Check sheet for the modelled part. Datum: model origin and axes. Units: mm. A direction names the side the tool comes from. Give positions to 0.01 mm unless a question says otherwise; leave off trailing zeros. Write each loop counter-clockwise with the first axis right and the second up, starting at its lowest first coordinate (ties: lowest second). Pieces come first, ordered by that corner, then holes. Notation, with made-up numbers: (49.25, 11) -> (82.25, 11) arc R5 cw to (82.25, 19) -> close; hole circle Ø9 at (-3, 26). An arc over 180 degrees is marked (long way). Return JSON: item names as keys, results as strings.
from build123d import *

# Parameters (mm, degrees)
PLATE_SKETCH_W                 = 80
PLATE_SKETCH_H                 = 70
PLATE_EXTRUDE_DEPTH            = 15
HOLE_CUT_REACH                 = 57.227
HOLE_SKETCH_R                  = 5.5
HOLE_CUT_DIRECTION_2_REACH     = 57.227
FEMALE_FILLET_RADIUS           = 7.5
FEMALE_FILLET_LENGTH           = 70
GAP_CUT_DEPTH                  = 10
GAP_CUT_DEPTH_BACK             = 10
GAP_SKETCH_W                   = 15
GAP_SKETCH_H                   = 15
PIN_SUPPORT_EXTRUDE_DEPTH      = 10
PIN_SUPPORT_EXTRUDE_DEPTH_BACK = 10
PIN_SUPPORT_SKETCH_W           = 15
PIN_SUPPORT_SKETCH_H           = 15
PIN_EXTRUDE_REACH              = 74.629
PIN_SKETCH_R                   = 5.5
PIN_EXTRUDE_DIRECTION_2_REACH  = 74.629
MALE_FILLET_RADIUS             = 7.5
MALE_FILLET_LENGTH             = 20


with BuildPart() as part:
    # Plate Sketch → Plate Extrude (new body)
    with BuildSketch(Plane.XY):
        Rectangle(PLATE_SKETCH_W, PLATE_SKETCH_H)
    extrude(amount=-PLATE_EXTRUDE_DEPTH)

    # Hole Cut: up to this face of the body (flat: up to its plane)
    hole_cut_end = Plane(part.part.faces().sort_by_distance((0, 35, -7.5))[0])
    # Hole Sketch → Hole Cut (cut, up to the picked face)
    with BuildSketch(Plane(origin=(0, 0, 0), x_dir=(1, 0, 0), z_dir=(0, 1, 0)), mode=Mode.PRIVATE) as hole_cut_sk1:
        with Locations(Location((-32.5, 7.5, 0), (0, 0, 90))):
            Circle(HOLE_SKETCH_R)
    hole_cut_tool1 = split(extrude(hole_cut_sk1.sketch, amount=HOLE_CUT_REACH, mode=Mode.PRIVATE), bisect_by=hole_cut_end, keep=Keep.BOTH, mode=Mode.PRIVATE)
    add(hole_cut_tool1.solids().sort_by(Axis((-32.5, 0, -7.5), (0, 1, 0)))[0], mode=Mode.SUBTRACT)

    # Hole Cut direction 2: up to this face of the body (flat: up to its plane)
    hole_cut_direction_2_end = Plane(part.part.faces().sort_by_distance((0, -35, -7.5))[0])
    # Hole Sketch → Hole Cut direction 2 (cut, up to the picked face)
    with BuildSketch(Plane(origin=(0, 0, 0), x_dir=(1, 0, 0), z_dir=(0, 1, 0)), mode=Mode.PRIVATE) as hole_cut_direction_2_sk1:
        with Locations(Location((-32.5, 7.5, 0), (0, 0, 90))):
            Circle(HOLE_SKETCH_R)
    hole_cut_direction_2_tool1 = split(extrude(hole_cut_direction_2_sk1.sketch, amount=-HOLE_CUT_DIRECTION_2_REACH, mode=Mode.PRIVATE), bisect_by=hole_cut_direction_2_end, keep=Keep.BOTH, mode=Mode.PRIVATE)
    add(hole_cut_direction_2_tool1.solids().sort_by(Axis((-32.5, 0, -7.5), (0, -1, 0)))[0], mode=Mode.SUBTRACT)

    # Female Fillet: full round fillet: the end face becomes a half cylinder, R = half its width
    female_fillet_face = Plane((-40, 0, -7.5), x_dir=(0, -1, 0), z_dir=(-1, 0, 0))  # on the end face: x along it, z out of the body
    female_fillet_slab = female_fillet_face.offset(-FEMALE_FILLET_RADIUS / 2) * Box(FEMALE_FILLET_LENGTH, 2 * FEMALE_FILLET_RADIUS, FEMALE_FILLET_RADIUS, mode=Mode.PRIVATE)  # the body's end, R deep
    female_fillet_round = Plane((-32.5, 0, -7.5), x_dir=(-1, 0, 0), z_dir=(0, -1, 0)) * Cylinder(FEMALE_FILLET_RADIUS, FEMALE_FILLET_LENGTH, mode=Mode.PRIVATE)  # its axis R under the face
    add(female_fillet_slab - female_fillet_round, mode=Mode.SUBTRACT)

    # Gap Sketch → Gap Cut (cut, two sides: drawn at the far end of the back side and taken through both)
    with BuildSketch(Plane(origin=(0, 0, 0), x_dir=(1, 0, 0), z_dir=(0, 1, 0)).offset(-GAP_CUT_DEPTH_BACK)):
        with Locations((-32.5, 7.5)):
            Rectangle(GAP_SKETCH_W, GAP_SKETCH_H)
    extrude(amount=GAP_CUT_DEPTH + GAP_CUT_DEPTH_BACK, mode=Mode.SUBTRACT)

    # Pin Support Sketch → Pin Support Extrude (add, two sides: drawn at the far end of the back side and taken through both)
    with BuildSketch(Plane(origin=(0, 0, 0), x_dir=(1, 0, 0), z_dir=(0, 1, 0)).offset(-PIN_SUPPORT_EXTRUDE_DEPTH_BACK)):
        with Locations((47.5, 7.5)):
            Rectangle(PIN_SUPPORT_SKETCH_W, PIN_SUPPORT_SKETCH_H)
    extrude(amount=PIN_SUPPORT_EXTRUDE_DEPTH + PIN_SUPPORT_EXTRUDE_DEPTH_BACK)

    # Pin Extrude: up to this face of the body (flat: up to its plane)
    pin_extrude_end = Plane(part.part.faces().sort_by_distance((3.713685867, 35, -7.5))[0])
    # Pin Sketch → Pin Extrude (add, up to the picked face)
    with BuildSketch(Plane(origin=(0, 10, 0), x_dir=(1, 0, 0), z_dir=(0, 1, 0)), mode=Mode.PRIVATE) as pin_extrude_sk1:
        with Locations(Location((47.5, 7.5, 0), (0, 0, 90))):
            Circle(PIN_SKETCH_R)
    pin_extrude_tool1 = split(extrude(pin_extrude_sk1.sketch, amount=PIN_EXTRUDE_REACH, mode=Mode.PRIVATE), bisect_by=pin_extrude_end, keep=Keep.BOTH, mode=Mode.PRIVATE)
    add(pin_extrude_tool1.solids().sort_by(Axis((47.5, 10, -7.5), (0, 1, 0)))[0])

    # Pin Extrude direction 2: up to this face of the body (flat: up to its plane)
    pin_extrude_direction_2_end = Plane(part.part.faces().sort_by_distance((3.713685867, -35, -7.5))[0])
    # Pin Sketch → Pin Extrude direction 2 (add, up to the picked face)
    with BuildSketch(Plane(origin=(0, 10, 0), x_dir=(1, 0, 0), z_dir=(0, 1, 0)), mode=Mode.PRIVATE) as pin_extrude_direction_2_sk1:
        with Locations(Location((47.5, 7.5, 0), (0, 0, 90))):
            Circle(PIN_SKETCH_R)
    pin_extrude_direction_2_tool1 = split(extrude(pin_extrude_direction_2_sk1.sketch, amount=-PIN_EXTRUDE_DIRECTION_2_REACH, mode=Mode.PRIVATE), bisect_by=pin_extrude_direction_2_end, keep=Keep.BOTH, mode=Mode.PRIVATE)
    add(pin_extrude_direction_2_tool1.solids().sort_by(Axis((47.5, 10, -7.5), (0, -1, 0)))[0])

    # Male Fillet: full round fillet: the end face becomes a half cylinder, R = half its width
    male_fillet_face = Plane((55, 0, -7.5), x_dir=(0, 1, 0), z_dir=(1, 0, 0))  # on the end face: x along it, z out of the body
    male_fillet_slab = male_fillet_face.offset(-MALE_FILLET_RADIUS / 2) * Box(MALE_FILLET_LENGTH, 2 * MALE_FILLET_RADIUS, MALE_FILLET_RADIUS, mode=Mode.PRIVATE)  # the body's end, R deep
    male_fillet_round = Plane((47.5, 0, -7.5), x_dir=(1, 0, 0), z_dir=(0, 1, 0)) * Cylinder(MALE_FILLET_RADIUS, MALE_FILLET_LENGTH, mode=Mode.PRIVATE)  # its axis R under the face
    add(male_fillet_slab - male_fillet_round, mode=Mode.SUBTRACT)


solid = part.part
(1) Set-up check for faces 4 (the flat face through (40, 22, -7)), 5 (the cylindrical face through (42.047, 22.325, -6.784)), 6 (the cylindrical face through (42.047, -22.325, -6.784)): record each of +Z, -Z, +X, -X, +Y, -Y from which the full face is reachable in a straight line by a thin tool's end or side.
Reply:
{"face 4": "+Z, -Z, +Y", "face 5": "+Y", "face 6": "-Y"}
(2) Cross-section at C-C on x = -34. Enter the section's corners in (y, z), then the cut area to 3 significant figures.
Reply:
{"outline": "(-35, -14.85) -> (-10, -14.85) -> (-10, -12.79) -> (-35, -12.79) -> close; (-35, -2.21) -> (-10, -2.21) -> (-10, -0.15) -> (-35, -0.15) -> close; (10, -14.85) -> (35, -14.85) -> (35, -12.79) -> (10, -12.79) -> close; (10, -2.21) -> (35, -2.21) -> (35, -0.15) -> (10, -0.15) -> close", "area": "206 mm^2"}
(3) Cross-section at A-A on y = 13. Enter the section's corners in (x, z), then the cut area to 3 significant figures.
Reply:
{"outline": "(-32.5, -15) -> (40, -15) -> (40, 0) -> (-32.5, 0) arc R7.5 ccw to start; circle Ø11 at (47.5, -7.5); hole circle Ø11 at (-32.5, -7.5)", "area": "1,180 mm^2"}
(4) Depth check by flat-ended pin: pin 1 Ø7.5 at (y, z) = (22, -8) entering from +X; pin 2 Ø1.5 at (y, z) = (-5.5, -3.5) entering from -X. Enter the tip coordinate at first touch or a pass-through.
Reply:
{"pin 1": "x = 53", "pin 2": "x = -25"}
(5) Thickness scan on L1, parallel to X at y = -15, z = -7.5; L2, parallel to Z at x = -32.5, y = -24.75; L3, parallel to X at y = 29, z = -6.75. Record the ranges inside material, lowest first.
Reply:
{"L1": "-40 to -38, -27 to 40, 42 to 53", "L2": "-15 to -13, -2 to 0", "L3": "-39.96 to -37.95, -27.05 to 40, 42.05 to 52.95"}
(6) Cross-section at B-B on z = -7.5. Enter the section's corners in (x, y), then the cut area to 3 significant figures.
Reply:
{"outline": "(-40, -35) -> (-38, -35) -> (-38, -10) -> (-40, -10) -> close; (-40, 10) -> (-38, 10) -> (-38, 35) -> (-40, 35) -> close; (-27, -35) -> (40, -35) -> (40, -10) -> (42, -10) -> (42, -35) -> (53, -35) -> (53, -10) -> (55, -10) -> (55, 10) -> (53, 10) -> (53, 35) -> (42, 35) -> (42, 10) -> (40, 10) -> (40, 35) -> (-27, 35) -> (-27, 10) -> (-25, 10) -> (-25, -10) -> (-27, -10) -> close", "area": "5,600 mm^2"}
(7) Release check for a two-part mould opening along Y. For faces 1 (the flat face through (-28, 10, -4)), 2 (the flat face through (7, 0, 0)), 3 (the flat face through (-1, 35, -7)) record: pulls with the +Y half, pulls with the -Y half, needs draft (parallel to the pull), parting line crosses it, or undercut.
Reply:
{"face 1": "undercut", "face 2": "needs draft", "face 3": "pulls with the +Y half"}
